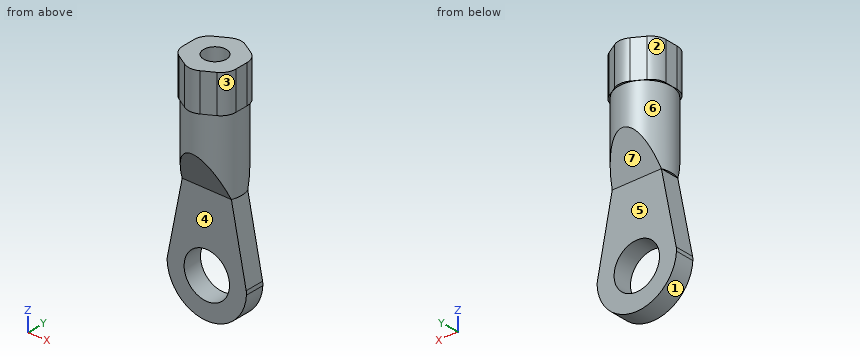
```python
from build123d import *

# Parameters (mm, degrees)
EXTRUDE_1_DEPTH          = 2.5
SKETCH_2_R               = 3
CUT_EXTRUDE_1_DEPTH      = 2.5
FILLET_1_R               = 2
SKETCH_3_R               = 3.482097069
EXTRUDE_2_DEPTH          = 15
CUT_EXTRUDE_2_DEPTH      = 15
CUT_EXTRUDE_2_DEPTH_BACK = 15
SKETCH_6_R               = 1.5
CUT_EXTRUDE_3_DEPTH      = 10
EXTRUDE_3_DEPTH          = 5
SKETCH_8_R               = 1.5
CUT_EXTRUDE_4_DEPTH      = 5
FILLET_2_R               = 2


with BuildPart() as part:
    # Sketch 1 → Extrude 1 (new body)
    with BuildSketch(Plane(origin=(0, 0, 0), x_dir=(1, 0, 0), z_dir=(0, 1, 0))):
        with BuildLine():
            ThreePointArc((5.25, 0), (0, 5.25), (-5.25, 0))
            Line((-5.25, 0), (-3.25, -10))
            Line((-3.25, -10), (3.25, -10))
            Line((3.25, -10), (5.25, 0))
        make_face()
    extrude(amount=EXTRUDE_1_DEPTH)

    # Sketch 2 → Cut-Extrude 1 (cut)
    with BuildSketch(Plane(origin=(0, 2.5, 0), x_dir=(1, 0, 0), z_dir=(0, 1, 0))):
        with Locations(Location((0, 0, 0), (0, 0, 270))):
            Circle(SKETCH_2_R)
    extrude(amount=-CUT_EXTRUDE_1_DEPTH, mode=Mode.SUBTRACT)

    # Fillet 1
    fillet_1_edges = [part.edges().sort_by_distance(p)[0] for p in [
        (-5.25, 1.25, 0),
        (5.25, 1.25, 0),
    ]]
    fillet(fillet_1_edges, radius=FILLET_1_R)

    # Sketch 3 → Extrude 2 (add)
    with BuildSketch(Plane.XY.offset(10)):
        with Locations(Location((0, 1.25, 0), (0, 0, 158.962488975))):
            Circle(SKETCH_3_R)
    extrude(amount=EXTRUDE_2_DEPTH)

    # Sketch 5 → Cut-Extrude 2 (cut, two sides: drawn at the far end of the back side and taken through both)
    with BuildSketch(Plane(origin=(0, 0, 0), x_dir=(0, 0, -1), z_dir=(1, 0, 0)).offset(-CUT_EXTRUDE_2_DEPTH_BACK)):
        Polygon((-10, 2.5), (-15, 4.732097069), (-10, 4.732097069), align=None)
        Polygon((-10, 0), (-15, -2.232097069), (-10, -2.232097069), align=None)
    extrude(amount=CUT_EXTRUDE_2_DEPTH + CUT_EXTRUDE_2_DEPTH_BACK, mode=Mode.SUBTRACT)

    # Sketch 6 → Cut-Extrude 3 (cut)
    with BuildSketch(Plane.XY.offset(25)):
        with Locations((0, 1.25)):
            Circle(SKETCH_6_R)
    extrude(amount=-CUT_EXTRUDE_3_DEPTH, mode=Mode.SUBTRACT)

    # Sketch 7 → Extrude 3 (add)
    with BuildSketch(Plane.XY.offset(25)):
        Polygon((0, 5.291451884), (-3.5, 3.270725942), (-3.5, -0.770725942), (0, -2.791451884), (3.5, -0.770725942), (3.5, 3.270725942), align=None)
    extrude(amount=-EXTRUDE_3_DEPTH)

    # Sketch 8 → Cut-Extrude 4 (cut)
    with BuildSketch(Plane.XY.offset(25)):
        with Locations((0, 1.25)):
            Circle(SKETCH_8_R)
    extrude(amount=-CUT_EXTRUDE_4_DEPTH, mode=Mode.SUBTRACT)

    # Fillet 2
    fillet_2_edges = [part.edges().sort_by_distance(p)[0] for p in [
        (0, 5.291451884, 22.5),
        (3.5, 3.270725942, 22.5),
        (3.5, -0.770725942, 22.5),
        (0, -2.791451884, 22.5),
        (-3.5, -0.770725942, 22.5),
        (-3.5, 3.270725942, 22.5),
    ]]
    fillet(fillet_2_edges, radius=FILLET_2_R)


solid = part.part
```
Can you work these out from the model? Positions are in its coordinate system, mm. Face numbers are marked on the shaded views. A direction names the side the tool comes from. Coordinates: 2 decimals unless noted, no trailing zeros. Order: outer loops, then holes, each group sorted by start corner. A loop starts at its lowest first (then second) coordinate and runs counter-clockwise, first axis right, second up. Notation, with made-up numbers: (29, 72.25) - (40, 72.25) arc R8 cw to (40, 79.25) - close; hole circle Ø2 at (2, 47.25). An arc over 180 degrees is marked (long way). Answer in a Markdown table with one row per item.
1. Suppose I cut it at C-C (y = 3.5). Please give me the cut outline in (x, z), and give its area (3 significant figures).
Reply:
| item | result |
|---|---|
| outline | (-2.94, 20) - (-2.66, 20) - (-2.66, 12.24) - (2.66, 12.24) - (2.66, 20) - (2.94, 20) - (2.94, 25) - (-2.94, 25) - close |
| area | 70.7 mm^2 |
2. Suppose I cut it at B-B (z = 19). Please give me the cut outline in (x, y).
Reply:
| item | result |
|---|---|
| outline | circle Ø6.96 at (0, 1.25); hole circle Ø3 at (0, 1.25) |
3. If we mould it in two halves opening along Z, with no side actions, what happens to the marked faces 5, 6 and 7? For each: pulls with the +Z half, pulls with the -Z half, needs draft (parallel to the pull), parting line crosses it, or undercut.
Reply:
| item | result |
|---|---|
| face 5 | needs draft |
| face 6 | undercut |
| face 7 | pulls with the -Z half |
4. If I drill on line 1 along Y through (x, z) = (0, 20.5); line 2 along Z through (x, y) = (3, -0.75); line 3 along Y through (x, z) = (0.5, 16.5), over which ranges is the centre line in solid material (lowest first)?
Reply:
| item | result |
|---|---|
| line 1 | y = -2.48 to -0.25, 2.75 to 4.98 |
| line 2 | z = 20 to 25 |
| line 3 | y = -2.2 to -0.16, 2.66 to 4.7 |
5. Suppose I cut it at D-D (z = 8). Please give me the cut outline in (x, y).
Reply:
| item | result |
|---|---|
| outline | (-3.65, 0) - (3.65, 0) - (3.65, 2.5) - (-3.65, 2.5) - close |
6. For pin 1 (1.4 mm diameter, centred on y = 1.5, z = 23.5, fed in from -X); pin 2 (2 mm diameter, centred on x = 3, y = 2, fed in from -Z); pin 3 (1.5 mm diameter, centred on y = -1.5, z = 21, fed in from -X), each with a flat end and sliding along its axis, tell me the tip position at first contact or that it passes through.
Reply:
| item | result |
|---|---|
| pin 1 | stops at x = -3.5 |
| pin 2 | stops at z = -4.85 |
| pin 3 | stops at x = -3.15 |
7. For the marked faces 1, 2, 3 and 4, which set-ups out of +Z, -Z, +X, -X, +Y, -Y let a thin tool reach every point of the face, with its end or its side?
Reply:
| item | result |
|---|---|
| face 1 | -Z, +Y, -Y |
| face 2 | +Z, -X, +Y |
| face 3 | +Z, +X, -Y |
| face 4 | -Z, +X, -X, -Y |
